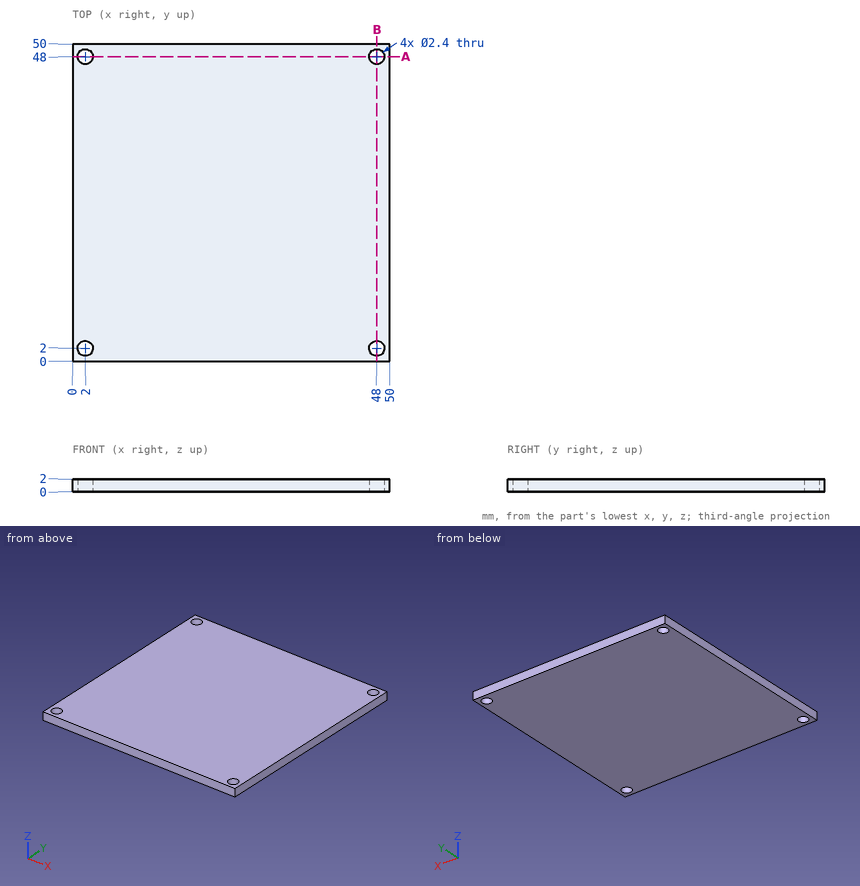
Geometry check sheet. Reference: drawing and pictorial views, mm from the part's lowest x, y, z. Coordinates: 2 decimals unless noted, no trailing zeros. Write each loop counter-clockwise with the first axis right and the second up, starting at its lowest first coordinate (ties: lowest second). Pieces come first, ordered by that corner, then holes.
Item 1: Depth check by flat-ended pin: pin 1 Ø2 at (x, y) = (48, 48) entering from -Z. Enter the tip coordinate at first touch or a pass-through.
Numbers:
pin 1: passes through
Item 2: Scan lines: probe 1 along Y at (x, z) = (2, 0.65); probe 2 along X at (y, z) = (2.5, 0.3). Record each from-to range of solid material in increasing order.
Numbers:
probe 1: y = 0 to 0.8, 3.2 to 46.8, 49.2 to 50
probe 2: x = 0 to 0.91, 3.09 to 46.91, 49.09 to 50
Item 3: Cross-section at A-A on y = 48. Record the boundary of the cut face in (x, z).
Numbers:
outline: (0, 0) - (0.8, 0) - (0.8, 2) - (0, 2) - close; (3.2, 0) - (46.8, 0) - (46.8, 2) - (3.2, 2) - close; (49.2, 0) - (50, 0) - (50, 2) - (49.2, 2) - close
